from build123d import *

# Parameters (mm, degrees)
SKETCH2_W       = 31.75
SKETCH2_H       = 76.2
SKETCH2_R       = 4.0386
EXTRUDE1_DEPTH  = 6.35
EXTRUDE2_DEPTH  = 6.35
EXTRUDE3_START  = 3.175
SKETCH4_R       = 15.875
EXTRUDE3_DEPTH  = 3.175
RIB1_REACH      = 117.441
SKETCH6_WALLS_W = 6.35
SKETCH6_WALLS_H = 292.649439439
SKETCH7_R       = 4.7625
EXTRUDE4_DEPTH  = 107.729125594
FILLET1_R       = 3.175
FILLET2_R       = 6.35


with BuildPart() as part:
    # Sketch2 → Extrude1 (new body)
    with BuildSketch(Plane(origin=(0, 0, 0), x_dir=(1, 0, 0), z_dir=(0, 1, 0))):
        with Locations((15.875, 38.1)):
            Rectangle(SKETCH2_W, SKETCH2_H)
        with Locations(Location((12.7, 12.7, 0), (0, 0, 270))):
            Circle(SKETCH2_R, mode=Mode.SUBTRACT)
        with Locations(Location((12.7, 63.5, 0), (0, 0, 90))):
            Circle(SKETCH2_R, mode=Mode.SUBTRACT)
    extrude(amount=-EXTRUDE1_DEPTH)

    # Sketch3 → Extrude2 (add)
    with BuildSketch(Plane(origin=(31.75, 0, 0), x_dir=(0, 0, -1), z_dir=(1, 0, 0))):
        with BuildLine():
            Line((9.525, 0), (66.675, 0))
            Line((66.675, 0), (53.680706216, 66.542567797))
            ThreePointArc((53.680706216, 66.542567797), (38.1, 79.375), (22.519293784, 66.542567797))
            Line((22.519293784, 66.542567797), (9.525, 0))
        make_face()
    extrude(amount=-EXTRUDE2_DEPTH)

    # Sketch4 → Extrude3 (add)
    with BuildSketch(Plane(origin=(31.75, 0, 0), x_dir=(0, 0, -1), z_dir=(1, 0, 0)).offset(EXTRUDE3_START)):
        with Locations((38.1, 63.5)):
            Circle(SKETCH4_R)
    extrude(amount=-EXTRUDE3_DEPTH)

    # Sketch6 walls → Rib1 (add, up to next)
    with BuildSketch(Plane(origin=(0, 0, 0), x_dir=(0, 0, 1), z_dir=(-0.9052035812190267, 0.42497820714508305, 0)), mode=Mode.PRIVATE) as rib1_sk1:
        with Locations((-38.1, 29.883885307)):
            Rectangle(SKETCH6_WALLS_W, SKETCH6_WALLS_H)
    rib1_tool1 = extrude(rib1_sk1.sketch, amount=-RIB1_REACH, mode=Mode.PRIVATE) - part.part
    add(rib1_tool1.solids().sort_by_distance((12.7, 27.051, -38.1))[0])

    # Sketch7 → Extrude4 (cut, through all)
    with BuildSketch(Plane(origin=(25.4, 0, -9.525), x_dir=(0, 0, 1), z_dir=(-1, 0, 0))):
        with Locations((-28.575, 63.5)):
            Circle(SKETCH7_R)
    extrude(amount=-EXTRUDE4_DEPTH, mode=Mode.SUBTRACT)

    # Fillet1
    fillet1_edges = [part.edges().sort_by_distance(p)[0] for p in [
        (28.575, 0, -66.675),
        (28.575, 0, -9.525),
        (25.4, 0, -22.225),
        (25.4, 27.051, -34.925),
        (12.7, 0, -34.925),
        (25.4, 27.051, -41.275),
        (12.7, 0, -41.275),
        (25.4, 0, -53.975),
    ]]
    fillet(fillet1_edges, radius=FILLET1_R)

    # Fillet2
    fillet2_edges = [part.edges().sort_by_distance(p)[0] for p in [
        (31.75, -3.175, -76.2),
        (31.75, -3.175, 0),
    ]]
    fillet(fillet2_edges, radius=FILLET2_R)


solid = part.part
Verification items for the finished model (mm, model axes). A direction names the side the tool comes from. Coordinates: 2 decimals unless noted, no trailing zeros. Write each loop counter-clockwise with the first axis right and the second up, starting at its lowest first coordinate (ties: lowest second). Pieces come first, ordered by that corner, then holes. Notation, with made-up numbers: M 88,-23 L 131,-23 A9 cw 131,-14 Z; hole C 55.25,-36.5 d3. An arc over 180 degrees is marked long. Use a Markdown table: item, result.
Q1. Go/stop test with flat-tipped pins: P1, Ø6, axis at x = 16, y = 25, coming from the +Z side (3 decimals); P2, Ø2, axis at y = 18, z = -36, coming from the -X side; P3, Ø12.5, axis at y = 63.5, z = -38.1, coming from the -X side. Record where each tip stops, or that it passes through.
Reply:
| item | result |
|---|---|
| P1 | stops at z = -34.925 |
| P2 | stops at x = 7.98 |
| P3 | stops at x = 25.4 |
Q2. Thickness scan on line 1 (X direction, y = -4.5, z = -63.5); line 2 (Y direction, x = 28, z = -38); line 3 (Y direction, x = 8, z = -23). Record the ranges inside material, lowest first.
Reply:
| item | result |
|---|---|
| line 1 | x = 0 to 8.66, 16.74 to 31.75 |
| line 2 | y = -6.35 to 58.74, 68.26 to 79.37 |
| line 3 | y = -6.35 to 0 |
Q3. Draft check along Y on faces 4 (the face through (28.59, 35, -16.36)), 5 (the face through (30.1, 68.22, -38.72)), 6 (the face through (14.25, -3.13, -67.23)). Enter one of: +Y half, -Y half, draft (parallel to the pull), parting line (faces both ways), or undercut.
Reply:
| item | result |
|---|---|
| face 4 | +Y half |
| face 5 | undercut |
| face 6 | draft |
Q4. Sectioned sample at A-A, the plane x = 12.7. Record the boundary of the cut face in (y, z) (3 decimals), plus the area to 3 significant figures.
Reply:
| item | result |
|---|---|
| outline | M -6.35,-76.2 L 0,-76.2 L 0,-67.539 L -6.35,-67.539 Z; M -6.35,-59.461 L 0,-59.461 L 0,-44.45 A3.175 cw 3.175,-41.275 L 27.051,-41.275 L 27.051,-34.925 L 3.175,-34.925 A3.175 cw 0,-31.75 L 0,-16.739 L -6.35,-16.739 Z; M -6.35,-8.661 L 0,-8.661 L 0,0 L -6.35,0 Z |
| area | 557 mm² |
Q5. Sectioned sample at C-C, the plane z = -63.5. Record the boundary of the cut face in (x, y) (3 decimals), plus the area to 3 significant figures.
Reply:
| item | result |
|---|---|
| outline | M 0,-6.35 L 8.661,-6.35 L 8.661,0 L 0,0 Z; M 16.739,-6.35 L 31.75,-6.35 L 31.75,16.259 L 25.4,16.259 L 25.4,3.175 A3.175 cw 22.225,0 L 16.739,0 Z |
| area | 256 mm² |
Q6. Set-up check for faces 1 (the face through (28, 0.7, -8.9)), 2 (the face through (24.495, 28.995, -42.23)), 3 (the face through (16, 17, -34.925)): record each of +Z, -Z, +X, -X, +Y, -Y from which the full face is reachable in a straight line by a thin tool's end or side.
Reply:
| item | result |
|---|---|
| face 1 | +Z, +X, -X, +Y |
| face 2 | -Z, -X, +Y |
| face 3 | +Z, -X, +Y |
